```python
from build123d import *

# Parameters (mm, degrees)
F3_DEPTH = 6.2
F4_COUNT = 3


with BuildPart() as f1:
    # F0 (on Front) → F1 (revolve)
    with BuildSketch(Plane.XZ):
        Polygon((0, 17.5), (0, 0), (3.1, 0), (3.8, 1.827984), (3.8, 6), (5.812653, 6), (5.812653, 7.5), (13, 7.5), (13, 17.5), align=None)
    revolve(axis=Axis((0, 0, 8.75), (0, 0, -1)))


with BuildPart() as f3:
    # F2 (on face) → F3 (new body)
    with BuildSketch(Plane.XY.offset(17.5)):
        with BuildLine():
            Line((-4, -3.1), (-4, 3.1))
            Line((-4, 3.1), (-12.624975, 3.1))
            ThreePointArc((-12.624975, 3.1), (-13, 0), (-12.624975, -3.1))
            Line((-12.624975, -3.1), (-4, -3.1))
        make_face()
    extrude(amount=-F3_DEPTH)


with BuildPart() as f4_1:
    # F4: instance of F3
    add(f3.part.rotate(Axis((0, 0, 17.5), (0, 0, -1)), 1 * 360 / F4_COUNT))


with BuildPart() as f4_2:
    # F4: instance of F3
    add(f3.part.rotate(Axis((0, 0, 17.5), (0, 0, -1)), 2 * 360 / F4_COUNT))


with BuildPart() as f1_1:
    add(f1.part)

    # F5: cut F3, F4_1, F4_2
    add(f3.part, mode=Mode.SUBTRACT)
    add(f4_1.part, mode=Mode.SUBTRACT)
    add(f4_2.part, mode=Mode.SUBTRACT)


solid = f1_1.part
```
Work out the finished part from the listing and answer in its coordinate system (mm). A direction names the side the tool comes from. Give positions to 0.01 mm unless a question says otherwise; leave off trailing zeros. Loops run counter-clockwise (first coordinate to the right, second up) from the corner with the lowest first, then second, coordinate; pieces in that order, holes last. Notation, with made-up numbers: M 83,42 L 92,42 A22 ccw 92,65 Z; hole C 48.5,-31.75 d1. An arc over 180 degrees is marked long. One line per item, written item: value. Start each with the question number.
1. Each of these flat-tipped pins is pushed along its axis until it touches: P1, Ø7, axis at x = -10, z = 14.5, coming from the +Y side; P2, Ø6, axis at y = 2.5, z = 3.5, coming from the -X side; P3, Ø3, axis at x = -6.5, y = -3.5, coming from the -Z side. Where does it stop, or does it pass through?
2. Find section B-B (z = 14.5). Give the vertices of the cut face in (x, y), and give its area (3 significant figures).
3. Find section C-C (x = 0). Give the vertices of the cut face in (y, z), and give its area (3 significant figures).
4. Find the intervals of material crossed by probe 1 along Y at (x, z) = (0, 3.75); probe 2 along Z at (x, y) = (2.25, 5.5); probe 3 along Z at (x, y) = (-5.25, -10.25), in increasing order.
5. Which of the six approach directions +Z, -Z, +X, -X, +Y, -Y give full straight-line access (tool end or side, diameter ignored) to faces 1 (the face through (2.04, -3.44, 14.44)), 2 (the face through (-8, -3.1, 14)), 3 (the face through (-6, 3, 7.5))?
6. Determine the mould class of faces 4 (the face through (6.87, -5.7, 14.44)), 5 (the face through (-8, 3.1, 14)), 6 (the face through (-4, 0, 14)), 7 (the face through (-3.796, -0.167, 3.943)) for opening direction X: released by +X, released by -X, zero draft, split by the parting line, or undercut.
7. Find section D-D (y = -8.5). Give the vertices of the cut face in (x, z), and give its area (3 significant figures).
8. Find section A-A (y = 0). Give the vertices of the cut face in (x, z).
Reported:
1. P1: stops at y = 11.26
1. P2: stops at x = -5.75
1. P3: stops at z = 7.5
2. outline: M -12.62,-3.1 A13 ccw 3.63,-12.48 L -0.68,-5.01 L 4.68,-1.91 L 9,-9.38 A13 ccw 9,9.38 L 4.68,1.91 L -0.68,5.01 L 3.63,12.48 A13 ccw -12.62,3.1 L -4,3.1 L -4,-3.1 Z
2. area: 366 mm²
3. outline: M -13,7.5 L -5.81,7.5 L -5.81,6 L -3.8,6 L -3.8,1.83 L -3.1,0 L 3.1,0 L 3.8,1.83 L 3.8,6 L 5.81,6 L 5.81,7.5 L 13,7.5 L 13,17.5 L 6.2,17.5 L 6.2,11.3 L 4.62,11.3 L 4.62,17.5 L -4.62,17.5 L -4.62,11.3 L -6.2,11.3 L -6.2,17.5 L -13,17.5 Z
3. area: 302 mm²
4. probe 1: y = -3.8 to 3.8
4. probe 2: z = 7.5 to 11.3
4. probe 3: z = 7.5 to 17.5
5. face 1: +Z
5. face 2: +Z, -X
5. face 3: -Z
6. face 4: undercut
6. face 5: zero draft
6. face 6: released by -X
6. face 7: split by the parting line
7. outline: M -9.84,7.5 L 9.84,7.5 L 9.84,17.5 L 8.49,17.5 L 8.49,11.3 L 1.33,11.3 L 1.33,17.5 L -9.84,17.5 Z
7. area: 152 mm²
8. outline: M -13,7.5 L -5.81,7.5 L -5.81,6 L -3.8,6 L -3.8,1.83 L -3.1,0 L 3.1,0 L 3.8,1.83 L 3.8,6 L 5.81,6 L 5.81,7.5 L 13,7.5 L 13,17.5 L -4,17.5 L -4,11.3 L -13,11.3 Z
